For this review, take the finished solid that the model builds, in its own axes (mm). A direction names the side the tool comes from. Coordinates: 2 decimals unless noted, no trailing zeros. Order: outer loops, then holes, each group sorted by start corner. A loop starts at its lowest first (then second) coordinate and runs counter-clockwise, first axis right, second up.
from build123d import *

# Parameters (mm, degrees)
CROQUIS1_W              = 10
CROQUIS1_H              = 10
CROQUIS1_W_2            = 30
CROQUIS1_H_2            = 25
SALIENTE_EXTRUIR1_DEPTH = 15
CROQUIS2_R              = 2
CORTAR_EXTRUIR1_DEPTH   = 30


with BuildPart() as part:
    # Croquis1 → Saliente-Extruir1 (new, symmetric)
    with BuildSketch(Plane.XY):
        with Locations((-20, -7.5)):
            Rectangle(CROQUIS1_W, CROQUIS1_H)
        Rectangle(CROQUIS1_W_2, CROQUIS1_H_2)
        with Locations((20, -7.5)):
            Rectangle(CROQUIS1_W, CROQUIS1_H)
    extrude(amount=SALIENTE_EXTRUIR1_DEPTH, both=True)

    # Croquis2 → Cortar-Extruir1 (cut)
    with BuildSketch(Plane(origin=(0, -2.5, 0), x_dir=(1, 0, 0), z_dir=(0, 1, 0))):
        with Locations(Location((-20, 0, 0), (0, 0, 180))):
            Circle(CROQUIS2_R)
        with Locations((20, 0)):
            Circle(CROQUIS2_R)
    extrude(amount=-CORTAR_EXTRUIR1_DEPTH, mode=Mode.SUBTRACT)


solid = part.part
1. Take a section at C-C, the plane y = -9.25. Give the boundary of the cut face in (x, z).
Answer below:
outline: (-25, -15) - (25, -15) - (25, 15) - (-25, 15) - close; hole circle Ø4 at (-20, 0); hole circle Ø4 at (20, 0)
2. The part is to be moulded in two halves that separate along X. For faces 4 (the face through (-25, -8, 0)), 5 (the face through (18.4, -7.4, 1.2)), 6 (the face through (0, 12.5, 0)), say which applies: +X half, -X half, draft (parallel to the pull), parting line (faces both ways), or undercut.
Answer below:
face 4: -X half
face 5: undercut
face 6: draft
3. Take a section at A-A, the plane x = -20. Give the boundary of the cut face in (y, z).
Answer below:
outline: (-12.5, -15) - (-2.5, -15) - (-2.5, -2) - (-12.5, -2) - close; (-12.5, 2) - (-2.5, 2) - (-2.5, 15) - (-12.5, 15) - close
4. To check wall thickness, follow L1, parallel to Z at x = 20, y = -9.25; L2, parallel to Y at x = -22, z = 5; L3, parallel to X at y = 7.25, z = 2. State the ranges of each line that lie inside material, in increasing order.
Answer below:
L1: z = -15 to -2, 2 to 15
L2: y = -12.5 to -2.5
L3: x = -15 to 15
5. Machinability: for faces 1 (the face through (-15, 5, 0)), 2 (the face through (15, 5, 0)), 3 (the face through (25, -8, 0)), which of the approach directions +Z, -Z, +X, -X, +Y, -Y give a long, thin tool a straight path to every point of the face, cutting with its end or side? Answer none if there is none.
Answer below:
face 1: +Z, -Z, -X, +Y
face 2: +Z, -Z, +X, +Y
face 3: +Z, -Z, +X, +Y, -Y
6. Clearance check with flat-ended pins moving along their axes: pin 1 Ø8 at (x, z) = (19.5, 6.5) entering from +Y; pin 2 Ø4.5 at (y, z) = (3, -3.5) entering from -X; pin 3 Ø1 at (x, y) = (16.5, 8.5) entering from +Z. State where each tip first meets the part, or that it passes through.
Answer below:
pin 1: stops at y = -2.5
pin 2: stops at x = -15
pin 3: passes through
7. Take a section at D-D, the plane z = -11.75. Give the boundary of the cut face in (x, y).
Answer below:
outline: (-25, -12.5) - (25, -12.5) - (25, -2.5) - (15, -2.5) - (15, 12.5) - (-15, 12.5) - (-15, -2.5) - (-25, -2.5) - close
8. Take a section at B-B, the plane z = 0. Give the boundary of the cut face in (x, y).
Answer below:
outline: (-25, -12.5) - (-22, -12.5) - (-22, -2.5) - (-25, -2.5) - close; (-18, -12.5) - (18, -12.5) - (18, -2.5) - (15, -2.5) - (15, 12.5) - (-15, 12.5) - (-15, -2.5) - (-18, -2.5) - close; (22, -12.5) - (25, -12.5) - (25, -2.5) - (22, -2.5) - close
